from build123d import *

# Parameters (mm, degrees)
CUT_EXTRUDE1_DEPTH = 3.96916


with BuildPart() as part:
    # Sketch1 → Revolve1 (revolve)
    with BuildSketch(Plane.XY):
        with BuildLine():
            Line((0, 32.3), (4.499259698, 32.3))
            ThreePointArc((4.499259698, 32.3), (4.840258878, 32.165676851), (4.998041723, 31.834878237))
            Line((4.998041723, 31.834878237), (5.483758073, 24.888810821))
            ThreePointArc((5.483758073, 24.888810821), (5.350652899, 24.512933404), (4.984976048, 24.353932584))
            Line((4.984976048, 24.353932584), (2.4768, 24.353932584))
            Line((2.4768, 24.353932584), (2.4768, 17.832081348))
            Line((2.4768, 17.832081348), (4.965517241, 17.832081348))
            Line((4.965517241, 17.832081348), (4.965517241, 12.36916))
            Line((4.965517241, 12.36916), (4, 12.36916))
            Line((4, 12.36916), (4, 11.86916))
            Line((4, 11.86916), (5, 11.86916))
            Line((5, 11.86916), (6, 11.402852342))
            Line((6, 11.402852342), (6, 8.366307658))
            Line((6, 8.366307658), (5, 7.9))
            Line((5, 7.9), (6.7, 7.9))
            Line((6.7, 7.9), (7.2, 7.4))
            Line((7.2, 7.4), (7.2, -7.4))
            Line((7.2, -7.4), (6.7, -7.9))
            Line((6.7, -7.9), (5.004037223, -7.9))
            Line((5.004037223, -7.9), (4.745792083, -15.295173238))
            Line((4.745792083, -15.295173238), (4.140965321, -15.9))
            Line((4.140965321, -15.9), (0, -15.9))
            Line((0, -15.9), (0, 32.3))
        make_face()
    revolve(axis=Axis((0, -15.9, 0), (0, 1, 0)))

    # Sketch2 → Cut-Extrude1 (cut)
    with BuildSketch(Plane(origin=(0, 11.86916, 0), x_dir=(1, 0, 0), z_dir=(0, 1, 0))):
        Polygon((-6.5, -3.75277675), (0, -7.505553499), (6.5, -3.75277675), (6.5, 3.75277675), (0, 7.505553499), (-6.5, 3.75277675), align=None)
        Polygon((-5, -2.886751346), (0, -5.773502692), (5, -2.886751346), (5, 2.886751346), (0, 5.773502692), (-5, 2.886751346), align=None, mode=Mode.SUBTRACT)
    extrude(amount=-CUT_EXTRUDE1_DEPTH, mode=Mode.SUBTRACT)

    # Sketch3 → Revolve2 (revolve)
    with BuildSketch(Plane.XY):
        Polygon((-26.9, 4), (0, 4), (0, 5.7744), (-10.4104, 5.7744), (-11.836, 7.2), (-23.683115991, 7.2), (-24.606421053, 6.9), (-24.606421053, 5.76), (-25.753210526, 5.76), (-25.753210526, 6.9), (-26.9, 6.9), align=None)
    revolve(axis=Axis((0, 0, 0), (-1, 0, 0)))


solid = part.part
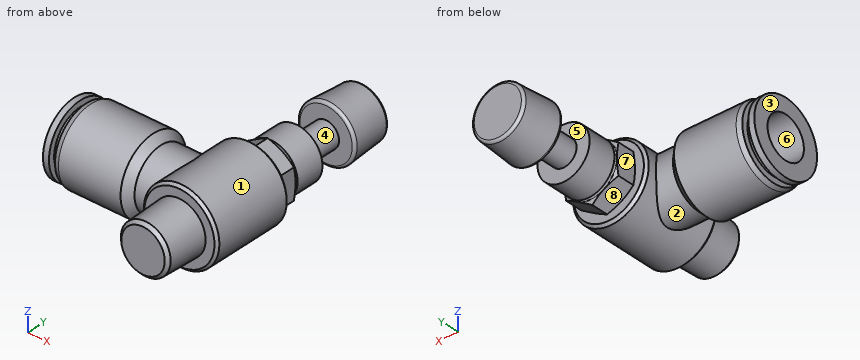
Input: part model. Units: mm. Frame: model coordinates. Face numbers are marked on the shaded views. A direction names the side the tool comes from. Coordinates: 2 decimals unless noted, no trailing zeros. Write each loop counter-clockwise with the first axis right and the second up, starting at its lowest first coordinate (ties: lowest second). Pieces come first, ordered by that corner, then holes. Notation, with made-up numbers: M 39,29.5 L 94,29.5 A12 cw 94,47.5 Z; hole C 33,82 d5. An arc over 180 degrees is marked long. Answer as a JSON object with one key per item and string values. Group by question number.
(1) Contact query for flat-ended pins moving along their axis: P1, Ø2, axis at y = 10, z = 0, coming from the -X side; P2, Ø4, axis at y = -0.5, z = -0.5, coming from the -X side; P3, Ø1, axis at y = 16.5, z = 1, coming from the +X side. Output: stop coordinate, or through.
(2) Mould query, pull axis X, two halves, no side actions, for the marked faces 1, 2, 3 and 4. Classes: pulls with the +X half, pulls with the -X half, needs draft (parallel to the pull), parting line crosses it, or undercut.
(3) Section B-B on x = -13.5. Output: boundary loops of the cut face in (y, z).
(4) Ray query, line 1 along Y through (x, z) = (-0.5, -4); line 2 along Z through (x, y) = (-22, 0). Return the intervals inside material, ascending. Write a range as [from, to].
(5) Section C-C on y = 22. Output: boundary loops of the cut face in (x, z).
(6) Section A-A on y = 0. Output: boundary loops of the cut face in (x, z), plus the area to 3 significant figures.
(7) Set-up query: the marked faces 5, 6, 7 and 8. Return all of +Z, -Z, +X, -X, +Y, -Y with unobstructed straight access to the full face (end or side cutting, diameter ignored); none if empty.
Result set:
{
 "1": {"P1": "stops at x = -5", "P2": "stops at x = -7.2", "P3": "stops at x = 4.94"},
 "2": {"face 1": "undercut", "face 2": "undercut", "face 3": "pulls with the -X half", "face 4": "parting line crosses it"},
 "3": {"outline": "C 0,0 d14.4; hole C 0,0 d8"},
 "4": {"line 1": "y = [-15.9, 11.87], [12.37, 17.83], [24.35, 32.3]", "line 2": "z = [-7.2, -4], [4, 7.2]"},
 "5": {"outline": "C 0,0 d4.95"},
 "6": {"outline": "M -26.9,-6.9 L -25.75,-6.9 L -25.75,-5.76 L -24.61,-5.76 L -24.61,-6.9 L -23.68,-7.2 L -11.84,-7.2 L -10.41,-5.77 L -4.3,-5.77 A7.2 ccw long -4.3,5.77 L -10.41,5.77 L -11.84,7.2 L -23.68,7.2 L -24.61,6.9 L -24.61,5.76 L -25.75,5.76 L -25.75,6.9 L -26.9,6.9 L -26.9,4 L -5.99,4 A7.2 ccw -5.99,-4 L -26.9,-4 Z", "area": "280 mm2"},
 "7": {"face 5": "none", "face 6": "-X", "face 7": "+Z, -Z, -X", "face 8": "-Z, -X"}
}
